For this review, take the finished solid that the model builds, in its own axes (mm). A direction names the side the tool comes from. Give positions to 0.01 mm unless a question says otherwise; leave off trailing zeros. Order: outer loops, then holes, each group sorted by start corner. A loop starts at its lowest first (then second) coordinate and runs counter-clockwise, first axis right, second up. Notation, with made-up numbers: (33, 58.25) - (51, 58.25) arc R12 ccw to (51, 66.25) - close; hole circle Ø4 at (-15.75, 27). An arc over 180 degrees is marked (long way). Put each result on its own line as item: value. Start each with the question number.
```python
from build123d import *

# Parameters (mm, degrees)
F6_DEPTH = 10
F7_START = -8
F7_DEPTH = 2
F9_R     = 2.5
F8_SIZE  = 0.4


with BuildPart() as f4:
    # F3 (on Front) → F4 (revolve)
    with BuildSketch(Plane.XZ):
        with BuildLine():
            ThreePointArc((-5, 21.8561575886), (-2.5645845405, 22.7103927734), (0, 23))
            Line((0, 23), (0, 26.8561575886))
            Line((0, 26.8561575886), (-5, 26.8561575886))
            Line((-5, 26.8561575886), (-5, 21.8561575886))
        make_face()
        with BuildLine():
            ThreePointArc((-5, 21.8561575886), (-11.2103927734, 8.9354154595), (0, 0))
            Line((0, 0), (0, 23))
            ThreePointArc((0, 23), (-2.5645845405, 22.7103927734), (-5, 21.8561575886))
        make_face()
    revolve(axis=Axis((0, 0, 13.4280787943), (0, 0, -1)))

    # F3 (on Front) → F5 (revolve)
    with BuildSketch(Plane.XZ):
        with BuildLine():
            ThreePointArc((-5, 21.8561575886), (-2.5645845405, 22.7103927734), (0, 23))
            Line((0, 23), (0, 26.8561575886))
            Line((0, 26.8561575886), (-5, 26.8561575886))
            Line((-5, 26.8561575886), (-5, 21.8561575886))
        make_face()
    revolve(axis=Axis((0, 0, 13.4280787943), (0, 0, -1)))

    # F3 (on Front) → F6 (join, symmetric)
    with BuildSketch(Plane.XZ):
        Polygon((0, 26.8561575886), (5, 26.8561575886), (10, 26.8561575886), (10, 36.8561575886), (5, 36.8561575886), (6.3397459622, 31.8561575886), (-6.3397459622, 31.8561575886), (-5, 36.8561575886), (-10, 36.8561575886), (-10, 26.8561575886), (-5, 26.8561575886), align=None)
    extrude(amount=F6_DEPTH, both=True)

    # F3 (on Front) → F7 (join)
    with BuildSketch(Plane.XZ.offset(F7_START)):
        Polygon((6.3397459622, 31.8561575886), (5, 36.8561575886), (-5, 36.8561575886), (-6.3397459622, 31.8561575886), align=None)
    extrude(amount=-F7_DEPTH)

    # F9
    f9_edges = [f4.edges().sort_by_distance(p)[0] for p in [
        (-5, 0, 24.356158),
        (5, 0, 21.856158),
        (5, 0, 26.856158),
    ]]
    fillet(f9_edges, radius=F9_R)

    # F8
    f8_edges = [f4.edges().sort_by_distance(p)[0] for p in [
        (0, -10, 26.856158),
        (10, -10, 31.856158),
        (7.5, -10, 36.856158),
        (5.669873, -10, 34.356158),
        (0, -10, 31.856158),
        (-5.669873, -10, 34.356158),
        (-7.5, -10, 36.856158),
        (-10, -10, 31.856158),
        (10, 0, 26.856158),
        (10, 10, 31.856158),
        (10, 0, 36.856158),
        (7.5, 0, 26.856158),
        (0, 10, 26.856158),
        (-10, 0, 26.856158),
        (-10, 0, 36.856158),
        (-10, 10, 31.856158),
        (0, 10, 36.856158),
    ]]
    chamfer(f8_edges, length=F8_SIZE)


solid = f4.part
```
1. Clearance check with flat-ended pins moving along their axes: pin 1 (1.5 mm diameter, centred on x = 0.5, z = 34, fed in from -Y); pin 2 (6.5 mm diameter, centred on x = 1.5, y = 1.5, fed in from +Z); pin 3 (3 mm diameter, centred on x = 5.5, z = 24, fed in from +Y). State where each tip first meets the part, or that it passes through.
2. Add section B-B, the plane z = 34.5. Give the boundary of the cut face in (x, y), then the cut area to 3 significant figures.
3. Add section C-C, the plane y = -8.25. Give the boundary of the cut face in (x, z), then the cut area to 3 significant figures.
4. Add section A-A, the plane y = 8.5. Give the boundary of the cut face in (x, z).
5. Wall thickness on line 1 (X direction, y = 7, z = 28); line 2 (Y direction, x = 0.75, z = 34.5); line 3 (Z direction, x = -3, y = -7.5): over which ranges is each line inside the solid? List them lowest first. Write a range as from..to.
6. Tool access review of faces 1 (the face through (5.66, -0.92, 34.39)), 2 (the face through (4, -7, 26.856)), 3 (the face through (0, 10, 32)): name each direction out of +Z, -Z, +X, -X, +Y, -Y from which nothing blocks a thin tool from reaching the whole face with its end or side.
7. The part is to be moulded in two halves that separate along X. For faces 4 (the face through (0, -10, 31)), 5 (the face through (-4.77, 1.5, 23.83)), 6 (the face through (0, -1, 31.856)), say which applies: released by +X, released by -X, zero draft, split by the parting line, or undercut.
8. Add section D-D, the plane z = 11.5. Give the boundary of the cut face in (x, y), then the cut area to 3 significant figures.
Found:
1. pin 1: stops at y = 8
1. pin 2: stops at z = 31.86
1. pin 3: stops at y = 3
2. outline: (-10, -9.6) - (-9.6, -10) - (-6.05, -10) - (-5.63, -9.6) - (-5.63, 8) - (5.63, 8) - (5.63, -9.6) - (6.05, -10) - (9.6, -10) - (10, -9.6) - (10, 9.6) - (9.6, 10) - (-9.6, 10) - (-10, 9.6) - close
2. area: 197 mm^2
3. outline: (-10, 27.26) - (-9.6, 26.86) - (9.6, 26.86) - (10, 27.26) - (10, 36.46) - (9.6, 36.86) - (5, 36.86) - (6.34, 31.86) - (-6.34, 31.86) - (-5, 36.86) - (-9.6, 36.86) - (-10, 36.46) - close; circle Ø16.02 at (0, 11.5)
3. area: 345 mm^2
4. outline: (-10, 27.26) - (-9.6, 26.86) - (9.6, 26.86) - (10, 27.26) - (10, 36.46) - (9.6, 36.86) - (-9.6, 36.86) - (-10, 36.46) - close; circle Ø15.49 at (0, 11.5)
5. line 1: x = -10..10
5. line 2: y = 8..10
5. line 3: z = 3.31..19.69, 26.86..31.86
6. face 1: -Y
6. face 2: none
6. face 3: +Z, +X, -X, +Y
7. face 4: zero draft
7. face 5: split by the parting line
7. face 6: undercut
8. outline: circle Ø23 at (0, 0)
8. area: 415 mm^2
